Model file for the job. Use its own axes, mm. Give positions to 0.01 mm unless a question says otherwise; leave off trailing zeros. Loops run counter-clockwise (first coordinate to the right, second up) from the corner with the lowest first, then second, coordinate; pieces in that order, holes last. Notation, with made-up numbers: M -26.5,-11.5 L 13.5,-11.5 A20 ccw 13.5,24.5 Z; hole C 55,57 d11. An arc over 180 degrees is marked long. Use CSV: the item, a comma, the result in double quotes. Start each with the question number.
(1) Flat gauge pins, fed straight in: P1, Ø0.9, axis at x = -1.5, y = 2, coming from the -Z side; P2, Ø1.5, axis at y = 1, z = 57.5, coming from the -X side; P3, Ø1.5, axis at x = -11, y = 2, coming from the +Z side. Where does each tip first touch, or does it go through?
(2) Slice it at C-C on z = 12. List the corners of the cut face in (x, y), and give its area (3 significant figures).
(3) Slice it at D-D on x = -14. List the corners of the cut face in (y, z), and give its area (3 significant figures).
(4) Slice it at B-B on z = 27.8. List the corners of the cut face in (x, y), and give its area (3 significant figures).
(5) Slice it at A-A on x = -10. List the corners of the cut face in (y, z).
(6) Wall check: line 1 along Z through (x, y) = (-5, 1.85); line 2 along X through (y, z) = (2.8, 22); line 3 along Z through (x, y) = (-9.75, 0.7). Give the ranges that are in metal, low to high. Write a range as from..to.
```python
from build123d import *

# Parameters (mm, degrees)
SKETCH_1_W          = 20
SKETCH_1_H          = 55.6
EXTRUDE_1_DEPTH     = 3
SKETCH_2_W          = 4
SKETCH_2_H          = 5
EXTRUDE_2_DEPTH     = 3
SKETCH_3_R          = 1.5
SKETCH_3_R_2        = 3
CUT_EXTRUDE_1_DEPTH = 10


with BuildPart() as part:
    # 草图1 → 凸台-拉伸1 (new body)
    with BuildSketch(Plane(origin=(0, 0, 0), x_dir=(1, 0, 0), z_dir=(0, 1, 0))):
        with Locations((-10, -27.8)):
            Rectangle(SKETCH_1_W, SKETCH_1_H)
    extrude(amount=EXTRUDE_1_DEPTH)

    # 草图2 → 凸台-拉伸2 (add)
    with BuildSketch(Plane(origin=(0, 3, 0), x_dir=(1, 0, 0), z_dir=(0, 1, 0))):
        with Locations((-14, 2.5)):
            Rectangle(SKETCH_2_W, SKETCH_2_H)
        with Locations((-6, 2.5)):
            Rectangle(SKETCH_2_W, SKETCH_2_H)
        with Locations((-14, -58.1)):
            Rectangle(SKETCH_2_W, SKETCH_2_H)
        with Locations((-6, -58.1)):
            Rectangle(SKETCH_2_W, SKETCH_2_H)
    extrude(amount=-EXTRUDE_2_DEPTH)

    # 草图3 → 切除-拉伸1 (cut)
    with BuildSketch(Plane(origin=(0, 3, 0), x_dir=(1, 0, 0), z_dir=(0, 1, 0))):
        with Locations(Location((-5.050252532, -22.850252532, 0), (0, 0, 270))):
            Circle(SKETCH_3_R)
        with Locations(Location((-10, -27.8, 0), (0, 0, 270))):
            Circle(SKETCH_3_R_2)
        with Locations(Location((-14.949747468, -32.749747468, 0), (0, 0, 270))):
            Circle(SKETCH_3_R)
        with Locations(Location((-5.050252532, -32.749747468, 0), (0, 0, 270))):
            Circle(SKETCH_3_R)
        with Locations(Location((-14.949747468, -22.850252532, 0), (0, 0, 270))):
            Circle(SKETCH_3_R)
        with Locations(Location((-14.949747468, -12.950757595, 0), (0, 0, 270))):
            Circle(SKETCH_3_R)
        with Locations(Location((-5.050252532, -12.950757595, 0), (0, 0, 270))):
            Circle(SKETCH_3_R)
        with Locations(Location((-14.949747468, -42.649242405, 0), (0, 0, 270))):
            Circle(SKETCH_3_R)
        with Locations(Location((-5.050252532, -42.649242405, 0), (0, 0, 270))):
            Circle(SKETCH_3_R)
    extrude(amount=-CUT_EXTRUDE_1_DEPTH, mode=Mode.SUBTRACT)


solid = part.part
```
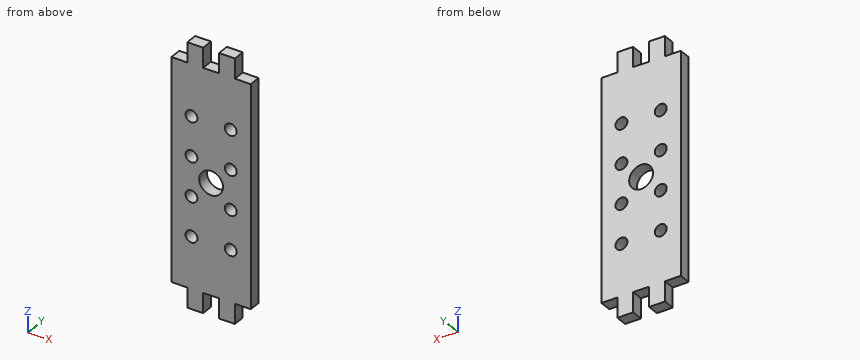
Reply:
1,P1,"stops at z = 0"
1,P2,"stops at x = -16"
1,P3,"stops at z = 55.6"
2,outline,"M -20,0 L -16.11,0 L -16.11,3 L -20,3 Z; M -13.79,0 L -6.21,0 L -6.21,3 L -13.79,3 Z; M -3.89,0 L 0,0 L 0,3 L -3.89,3 Z"
2,area,"46.1 mm^2"
3,outline,"M 0,-5 L 3,-5 L 3,11.79 L 0,11.79 Z; M 0,14.11 L 3,14.11 L 3,21.69 L 0,21.69 Z; M 0,24.01 L 3,24.01 L 3,31.59 L 0,31.59 Z; M 0,33.91 L 3,33.91 L 3,41.49 L 0,41.49 Z; M 0,43.81 L 3,43.81 L 3,60.6 L 0,60.6 Z"
3,area,"169 mm^2"
4,outline,"M -20,0 L -13,0 L -13,3 L -20,3 Z; M -7,0 L 0,0 L 0,3 L -7,3 Z"
4,area,"42.0 mm^2"
5,outline,"M 0,0 L 3,0 L 3,24.8 L 0,24.8 Z; M 0,30.8 L 3,30.8 L 3,55.6 L 0,55.6 Z"
6,line 1,"z = -5..11.45, 14.45..21.35, 24.35..31.25, 34.25..41.15, 44.15..60.6"
6,line 2,"x = -20..-16.19, -13.71..-6.29, -3.81..0"
6,line 3,"z = 0..24.81, 30.79..55.6"
